Verification items for the finished model (mm, model axes). Coordinates: 2 decimals unless noted, no trailing zeros. Write each loop counter-clockwise with the first axis right and the second up, starting at its lowest first coordinate (ties: lowest second). Pieces come first, ordered by that corner, then holes. Notation, with made-up numbers: M -4,-26.5 L 30,-26.5 A29 ccw 30,10.5 Z; hole C 5,27.25 d11. An arc over 180 degrees is marked long. Answer in a Markdown table with one row per item.
from build123d import *

# Parameters (mm, degrees)
CYLINDER001_R     = 1.5
CYLINDER001_DEPTH = 10
ARRAY001_X_COUNT  = 2
ARRAY001_X_PITCH  = 66
ARRAY001_Y_COUNT  = 2
ARRAY001_Y_PITCH  = 16
BOX002_W          = 76
BOX002_H          = 28
BOX002_DEPTH      = 0.5
FILLET001_R       = 5


with BuildPart() as screw_body_hole_array:
    # Cylinder001 → Cylinder001 (new body)
    with BuildSketch(Plane.XY):
        Circle(CYLINDER001_R)
    extrude(amount=CYLINDER001_DEPTH)

    # Array001 X: screw body hole array ×2


with BuildPart() as screw_body_hole_array_1:
    add(screw_body_hole_array.part)
    with Locations(*[(i * ARRAY001_X_PITCH, 0, 0) for i in range(1, ARRAY001_X_COUNT)]):
        add(screw_body_hole_array.part)

    # Array001 Y: screw body hole array ×2


with BuildPart() as screw_body_hole_array_2:
    add(screw_body_hole_array_1.part)
    with Locations(*[(0, i * ARRAY001_Y_PITCH, 0) for i in range(1, ARRAY001_Y_COUNT)]):
        add(screw_body_hole_array_1.part)


with BuildPart() as screw_body_hole_array_3:
    # Array001 placement: moved
    add(screw_body_hole_array_2.part.moved(Location((-5, 5, -4))))


with BuildPart() as amplifier_lid_cut:
    # Box002 → Box002 (new body)
    with BuildSketch(Plane(origin=(-10, -1, -1), x_dir=(1, 0, 0), z_dir=(0, 0, 1))):
        with Locations((38, 14)):
            Rectangle(BOX002_W, BOX002_H)
    extrude(amount=BOX002_DEPTH)

    # Fillet001
    fillet001_edges = [amplifier_lid_cut.edges().sort_by_distance(p)[0] for p in [
        (-10, -1, -0.75),
        (-10, 27, -0.75),
        (66, -1, -0.75),
        (66, 27, -0.75),
    ]]
    fillet(fillet001_edges, radius=FILLET001_R)

    # Cut001: cut screw body hole array
    add(screw_body_hole_array_3.part, mode=Mode.SUBTRACT)


solid = amplifier_lid_cut.part
1) Thickness scan on L1, parallel to X at y = 5, z = -0.65; L2, parallel to Y at x = -5, z = -0.8; L3, parallel to X at y = 3.75, z = -0.6. Record the ranges inside material, lowest first. Write a range as [from, to].
Response values:
| item | result |
|---|---|
| L1 | x = [-10, -6.5], [-3.5, 59.5], [62.5, 66] |
| L2 | y = [-1, 3.5], [6.5, 19.5], [22.5, 27] |
| L3 | x = [-9.99, -5.83], [-4.17, 60.17], [61.83, 65.99] |
2) Release check for a two-part mould opening along X. For faces 1 (the face through (-8.57, 25.5, -0.75)), 2 (the face through (-5.195, 22.487, -0.753)), 3 (the face through (27, 13, -1)) record: +X half, -X half, draft (parallel to the pull), parting line (faces both ways), or undercut.
Response values:
| item | result |
|---|---|
| face 1 | -X half |
| face 2 | undercut |
| face 3 | draft |
3) Sectioned sample at A-A (y = 21). Record the cut outline in (x, z).
Response values:
| item | result |
|---|---|
| outline | M -10,-1 L -6.5,-1 L -6.5,-0.5 L -10,-0.5 Z; M -3.5,-1 L 59.5,-1 L 59.5,-0.5 L -3.5,-0.5 Z; M 62.5,-1 L 66,-1 L 66,-0.5 L 62.5,-0.5 Z |
4) Sectioned sample at B-B (z = -0.85). Record the cut outline in (x, y).
Response values:
| item | result |
|---|---|
| outline | M -10,4 A5 ccw -5,-1 L 61,-1 A5 ccw 66,4 L 66,22 A5 ccw 61,27 L -5,27 A5 ccw -10,22 Z; hole C -5,5 d3; hole C -5,21 d3; hole C 61,5 d3; hole C 61,21 d3 |
5) Depth check by flat-ended pin: pin 1 (2.5 mm diameter, centred on x = -5, y = 5, fed in from +Z); pin 2 (5 mm diameter, centred on x = -5, y = 21, fed in from -Z). Enter the tip coordinate at first touch or a pass-through.
Response values:
| item | result |
|---|---|
| pin 1 | passes through |
| pin 2 | stops at z = -1 |
